from build123d import *

# Parameters (mm, degrees)
SKETCH1_R           = 45
BOSS_EXTRUDE1_DEPTH = 3
SKETCH2_R           = 45
SKETCH2_R_2         = 43
BOSS_EXTRUDE2_DEPTH = 100
BOSS_EXTRUDE3_DEPTH = 5
SKETCH4_W           = 3
SKETCH4_H           = 1.5
CUT_EXTRUDE1_DEPTH  = 5
CHAMFER1_SIZE       = 0.6
CHAMFER2_SIZE       = 1


with BuildPart() as part:
    # Sketch1 → Boss-Extrude1 (new body)
    with BuildSketch(Plane(origin=(0, 0, 0), x_dir=(1, 0, 0), z_dir=(0, 1, 0))):
        with Locations(Location((0, 0, 0), (0, 0, 270))):
            Circle(SKETCH1_R)
    extrude(amount=BOSS_EXTRUDE1_DEPTH)

    # Sketch2 → Boss-Extrude2 (add)
    with BuildSketch(Plane(origin=(0, 3, 0), x_dir=(1, 0, 0), z_dir=(0, 1, 0))):
        with Locations(Location((0, 0, 0), (0, 0, 270))):
            Circle(SKETCH2_R)
        with Locations(Location((0, 0, 0), (0, 0, 270))):
            Circle(SKETCH2_R_2, mode=Mode.SUBTRACT)
    extrude(amount=BOSS_EXTRUDE2_DEPTH)

    # Sketch3 → Boss-Extrude3 (add)
    with BuildSketch(Plane(origin=(0, 3, 0), x_dir=(1, 0, 0), z_dir=(0, 1, 0))):
        with BuildLine():
            Line((-1.5, -15.176050211), (-1.5, -17.184658856))
            ThreePointArc((-1.5, -17.184658856), (0, 17.25), (1.5, -17.184658856))
            Line((1.5, -17.184658856), (1.5, -15.176050211))
            ThreePointArc((1.5, -15.176050211), (0, 15.25), (-1.5, -15.176050211))
        make_face()
    extrude(amount=BOSS_EXTRUDE3_DEPTH)

    # Sketch4 → Cut-Extrude1 (cut)
    with BuildSketch(Plane.XY.offset(45)):
        with Locations((0, 3.75)):
            Rectangle(SKETCH4_W, SKETCH4_H)
    extrude(amount=-CUT_EXTRUDE1_DEPTH, mode=Mode.SUBTRACT)

    # Chamfer1
    chamfer1_edges = [part.edges().sort_by_distance(p)[0] for p in [
        (0, 103, -43),
    ]]
    chamfer(chamfer1_edges, length=CHAMFER1_SIZE)

    # Chamfer2
    chamfer2_edges = [part.edges().sort_by_distance(p)[0] for p in [
        (0, 0, -45),
    ]]
    chamfer(chamfer2_edges, length=CHAMFER2_SIZE)


solid = part.part
Build history of the part. All positions in model axes, mm. A direction names the side the tool comes from. Give positions to 0.01 mm unless a question says otherwise; leave off trailing zeros. Loops run counter-clockwise (first coordinate to the right, second up) from the corner with the lowest first, then second, coordinate; pieces in that order, holes last. Notation, with made-up numbers: (8, 43) - (62, 43) arc R18 ccw to (62, 51) - close; hole circle Ø9 at (-3, -12.75). An arc over 180 degrees is marked (long way). Write item = value, one per line. Start each with the question number.
1) Band-saw the part on A-A on x = 0. Give the cut face in (y, z).
2) Band-saw the part on C-C on y = 74.5. Give the cut face in (x, z), plus the area to 3 significant figures.
3) Probe probe 1 along X at (y, z) = (6.3, 0); probe 2 along X at (y, z) = (48, 0); probe 3 along Y at (x, z) = (4, -40). List the from-to ranges inside material, lowest first. Write a range as from..to.
4) Drop flat-ended pins along their axis: pin 1 Ø3 at (y, z) = (14.5, 3.5) entering from -X; pin 2 Ø3 at (x, z) = (16, 20) entering from -Y; pin 3 Ø6 at (x, y) = (-10, 71.5) entering from -Z; pin 4 Ø2 at (x, y) = (-26.5, 76.5) entering from -Z. Give the stop position or say it passes through.
5) Pull direction X, two halves, no side cores. Call faces 3 (the cylindrical face through (-17.235, 51.286, 41.569)), 4 (the flat face through (-14, 8, -6.5)), 5 (the flat face through (24, 103, -37)): +X half, -X half, draft (parallel to the pull), parting line (faces both ways), or undercut.
6) Band-saw the part on B-B on z = 0. Give the cut face in (x, y), plus the area to 3 significant figures.
7) Tool access for faces 1 (the flat face through (1, 0, -1)), 2 (the cylindrical face through (29.061, 52.004, -31.693)): list every direction of +Z, -Z, +X, -X, +Y, -Y with a clear straight run to the whole face (end or side of a thin tool).
Final values:
q1.outline = (0, -44) - (1, -45) - (103, -45) - (103, -43.6) - (102.4, -43) - (3, -43) - (3, -17.25) - (8, -17.25) - (8, -15.25) - (3, -15.25) - (3, 45) - (1, 45) - (0, 44) - close; (4.5, 43) - (102.4, 43) - (103, 43.6) - (103, 45) - (4.5, 45) - close
q2.outline = circle Ø90 at (0, 0); hole circle Ø86 at (0, 0)
q2.area = 553 mm²
q3.probe_1 = -45..-43, -17.25..-15.25, 15.25..17.25, 43..45
q3.probe_2 = -45..-43, 43..45
q3.probe_3 = 0..3
q4.pin_1 = -44.96
q4.pin_2 = 0
q4.pin_3 = -44.45
q4.pin_4 = -37.08
q5.face_3 = parting line
q5.face_4 = undercut
q5.face_5 = draft
q6.outline = (-45, 1) - (-44, 0) - (44, 0) - (45, 1) - (45, 103) - (43.6, 103) - (43, 102.4) - (43, 3) - (17.25, 3) - (17.25, 8) - (15.25, 8) - (15.25, 3) - (-15.25, 3) - (-15.25, 8) - (-17.25, 8) - (-17.25, 3) - (-43, 3) - (-43, 102.4) - (-43.6, 103) - (-45, 103) - close
q6.area = 689 mm²
q7.face_1 = +Z, -Z, +X, -X, -Y
q7.face_2 = +Y
